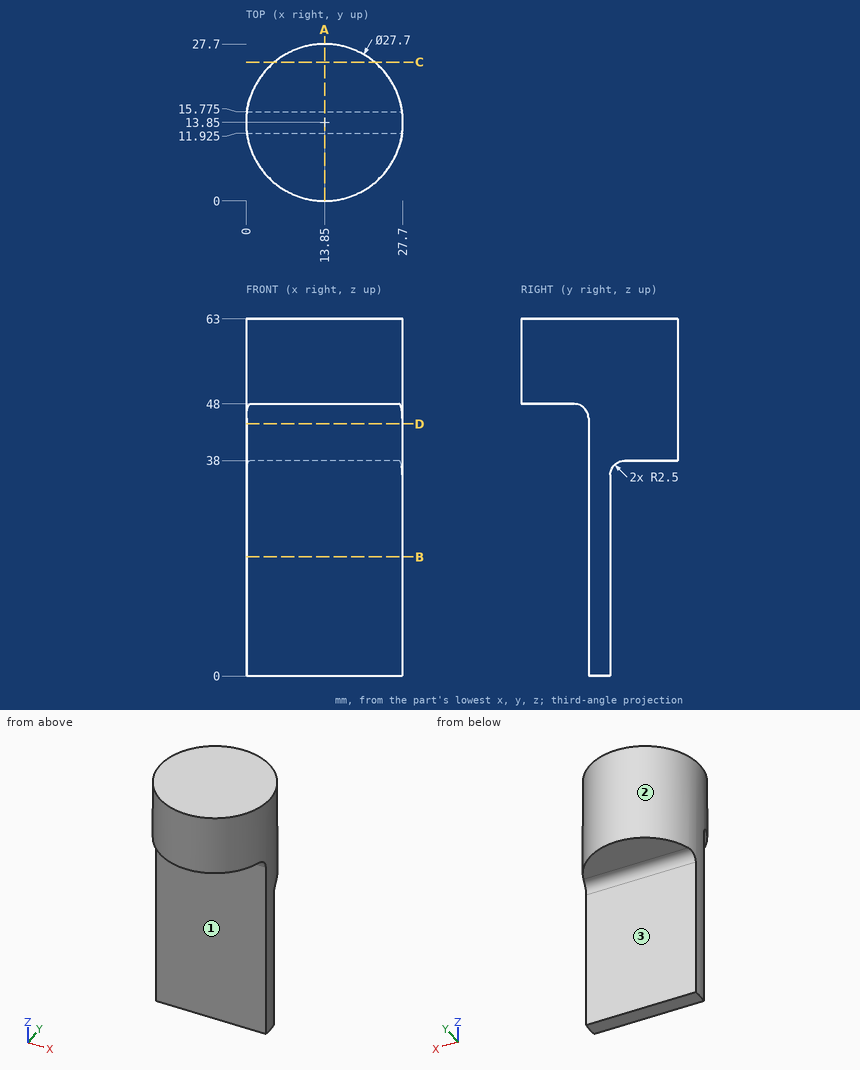
Geometry check sheet. Reference: drawing and pictorial views, mm from the part's lowest x, y, z. A direction names the side the tool comes from. Give positions to 0.01 mm unless a question says otherwise; leave off trailing zeros. Order: outer loops, then holes, each group sorted by start corner. A loop starts at its lowest first (then second) coordinate and runs counter-clockwise, first axis right, second up. Notation, with made-up numbers: (67.25, -23) - (97.25, -23) arc R24 cw to (97.25, 13) - close; hole circle Ø10 at (89.5, -1.5). An arc over 180 degrees is marked (long way). Use one line per item in the form item = value.
1) Access from +Z, -Z, +X, -X, +Y, -Y to the whole of each face (thin tool, end or side, straight path). Record for the marked faces 1, 2 and 3.
Working result:
face_1 = -Z, +X, -X, -Y
face_2 = +Z, -Z
face_3 = -Z, +X, -X, +Y
2) Material ranges on probe 1 along Y at (x, z) = (16.75, 29.5) (3 decimals); probe 2 along X at (y, z) = (14, 60.5); probe 3 along Z at (x, y) = (13.5, 9.5), recorded low to high. Write a range as from..to.
Working result:
probe_1 = 11.925..15.775
probe_2 = 0..27.7
probe_3 = 48..63
3) Sectioned sample at A-A (x = 13.85). Record the boundary of the cut face in (y, z) (3 decimals).
Working result:
outline = (0, 48) - (9.425, 48) arc R2.5 cw to (11.925, 45.5) - (11.925, 0) - (15.775, 0) - (15.775, 35.5) arc R2.5 cw to (18.275, 38) - (27.7, 38) - (27.7, 63) - (0, 63) - close
4) Sectioned sample at B-B (z = 21). Record the boundary of the cut face in (x, y) (3 decimals).
Working result:
outline = (0.134, 11.925) - (27.566, 11.925) arc R13.85 ccw to (27.566, 15.775) - (0.134, 15.775) arc R13.85 ccw to start
5) Sectioned sample at D-D (z = 44.5). Record the boundary of the cut face in (x, y) (3 decimals), and give its area (3 significant figures).
Working result:
outline = (0.134, 11.925) - (27.566, 11.925) arc R13.85 ccw (long way) to start
area = 354 mm^2
6) Depth check by flat-ended pin: pin 1 Ø5 at (y, z) = (8.5, 23) entering from -X; pin 2 Ø8 at (x, z) = (7.5, 25.5) entering from +Y (3 decimals); pin 3 Ø1.5 at (x, z) = (12.5, 42.5) entering from -Y (3 decimals); pin 4 Ø4.5 at (x, y) = (18.5, 6.5) entering from -Z. Enter the tip coordinate at first touch or a pass-through.
Working result:
pin_1 = through
pin_2 = 15.775
pin_3 = 11.925
pin_4 = 48
7) Sectioned sample at C-C (y = 24.5). Record the boundary of the cut face in (x, z).
Working result:
outline = (5, 38) - (22.7, 38) - (22.7, 63) - (5, 63) - close
